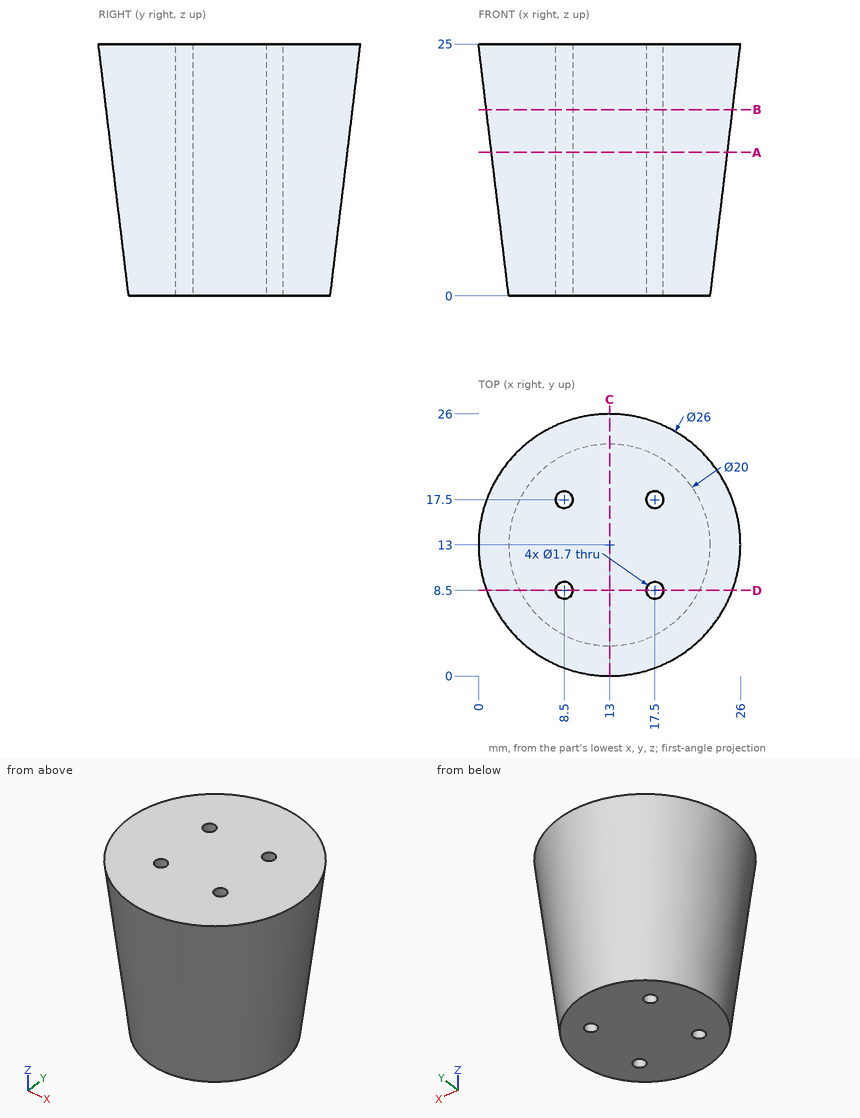
Check sheet for the drawn part. Datum: minimum x, y, z corner. Units: mm. Give positions to 0.01 mm unless a question says otherwise; leave off trailing zeros. Write each loop counter-clockwise with the first axis right and the second up, starting at its lowest first coordinate (ties: lowest second). Pieces come first, ordered by that corner, then holes. Notation, with made-up numbers: (16, 75.5) -> (60, 75.5) arc R10 ccw to (60, 88.5) -> close; hole circle Ø5 at (87.5, 1.25). An arc over 180 degrees is marked (long way). Use one line per item in the form item = value. Start each with the question number.
1. Section check D-D (y = 8.5). Count the separate pieces of the cut face and the enclosed holes in it, and give its area (3 significant figures).
2. Section check B-B (z = 18.5). Record the cut outline in (x, y).
3. Go/stop test with flat-tipped pins: P1, Ø5, axis at x = 12.5, z = 7.5, coming from the +Y side; P2, Ø2, axis at x = 4, z = 13.5, coming from the -Y side; P3, Ø1.5, axis at x = 7, z = 10, coming from the +Y side; P4, Ø1.5, axis at x = 8.5, y = 17.5, coming from the -Z side. Record where each tip stops, or that it passes through.
4. Section check A-A (z = 14.25). Record the cut outline in (x, y).
5. Section check C-C (x = 13). Record the cut outline in (y, z), and give its area (3 significant figures).
6. Thickness scan on line 1 along Y through (x, z) = (17.5, 8); line 2 along X through (y, z) = (17.5, 11); line 3 along Y through (x, z) = (17.5, 16). Record the ranges inside material, lowest first. Write a range as from..to.
Conclusion:
q1.separate_pieces = 3
q1.enclosed_holes = 0
q1.area = 444 mm²
q2.outline = circle Ø24.44 at (13, 13); hole circle Ø1.7 at (8.5, 8.5); hole circle Ø1.7 at (8.5, 17.5); hole circle Ø1.7 at (17.5, 8.5); hole circle Ø1.7 at (17.5, 17.5)
q3.P1 = 24.2
q3.P2 = 4.56
q3.P3 = 22.91
q3.P4 = through
q4.outline = circle Ø23.42 at (13, 13); hole circle Ø1.7 at (8.5, 8.5); hole circle Ø1.7 at (8.5, 17.5); hole circle Ø1.7 at (17.5, 8.5); hole circle Ø1.7 at (17.5, 17.5)
q5.outline = (0, 25) -> (3, 0) -> (23, 0) -> (26, 25) -> close
q5.area = 575 mm²
q6.line_1 = 3.01..7.65, 9.35..16.65, 18.35..22.99
q6.line_2 = 2.61..7.65, 9.35..16.65, 18.35..23.39
q6.line_3 = 1.96..7.65, 9.35..16.65, 18.35..24.04
